Work out the finished part from the listing and answer in its coordinate system (mm). Coordinates: 2 decimals unless noted, no trailing zeros. Loops run counter-clockwise (first coordinate to the right, second up) from the corner with the lowest first, then second, coordinate; pieces in that order, holes last. Notation, with made-up numbers: M 64.5,29.25 L 117.5,29.25 A17 ccw 117.5,39.25 Z; hole C 7.25,-22 d3. An arc over 180 degrees is marked long. Write each question's results on one line, items separated by ' | '.
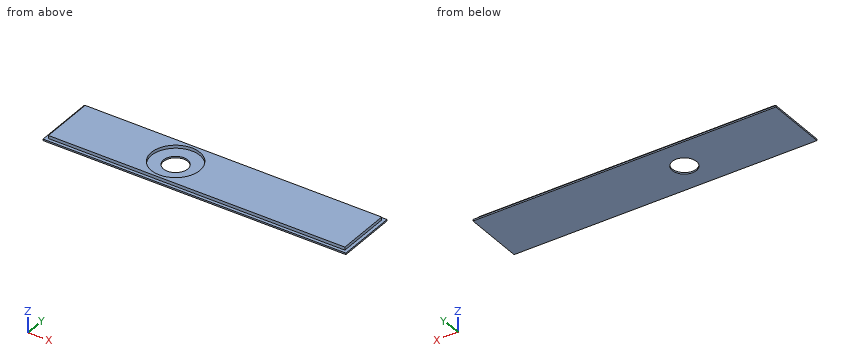
Autodesk Inventor part; units mm, degrees
ref_plane "YZ Plane" through (0, 0, 0) normal (1, 0, 0) x (0, 1, 0)
ref_plane "XZ Plane" through (0, 0, 0) normal (0, 1, 0) x (-1, 0, 0)
ref_plane "XY Plane" through (0, 0, 0) normal (0, 0, 1) x (1, 0, 0)
sketch "Boceto1" plane through (0, 0, 0) normal (0, 0, 1) x (1, 0, 0)
  line L0 (0, 0) -> (200, 0)
  line L1 (200, 0) -> (200, 40)
  line L2 (200, 40) -> (0, 40)
  line L3 (0, 40) -> (0, 0)
  circle A0 centre (74, 20) radius 8
  dimension "d0" = 200
  dimension "d1" = 40
  dimension "d2" = 16
  dimension "d3" = 74
  dimension "d4" = 20
extrude "Extrusión1" add sketch "Boceto1" along normal blind 1
sketch "Boceto2" plane through (0, 0, 1) normal (0, 0, 1) x (1, 0, 0)
  circle A0 centre (74, 20) radius 8
  line L0 (0, 0) -> (0, 40)
  line L1 (200, 0) -> (0, 0)
  line L2 (200, 40) -> (200, 0)
  line L3 (0, 40) -> (200, 40)
  line L4 (197.9, 37.9) -> (197.9, 2.1)
  line L5 (197.9, 2.1) -> (2.1, 2.1)
  line L6 (2.1, 2.1) -> (2.1, 37.9)
  line L7 (2.1, 37.9) -> (197.9, 37.9)
  circle A1 centre (74, 20) radius 16
  dimension "d7" = 2.1
  dimension "d8" = 32
extrude "Extrusión2" add sketch "Boceto2" along normal blind 2 contours L4 L5 L6 L7
properties part number "Tapa"
1) Straight lines are drawn through the part: probe 1 along Y at (x, z) = (74, 0.7); probe 2 along X at (y, z) = (20.5, 0.1); probe 3 along Y at (x, z) = (96.5, 2.7). For each, find the intervals that lie inside material, in ascending order. Write a range as [from, to].
Check result:
probe 1: [0, 12], [28, 40] | probe 2: [0, 66.02], [81.98, 200] | probe 3: [2.1, 37.9]
2) Find section D-D, the plane x = 105.5. Give the vertices of the cut face in (y, z), and give its area (3 significant figures).
Check result:
outline: M 0,0 L 40,0 L 40,1 L 37.9,1 L 37.9,3 L 2.1,3 L 2.1,1 L 0,1 Z | area: 112 mm^2
3) Find section A-A, the plane x = 74. Give the vertices of the cut face in (y, z).
Check result:
outline: M 0,0 L 12,0 L 12,1 L 4,1 L 4,3 L 2.1,3 L 2.1,1 L 0,1 Z; M 28,0 L 40,0 L 40,1 L 37.9,1 L 37.9,3 L 36,3 L 36,1 L 28,1 Z
4) Given pin 1 Ø2 at (x, y) = (77, 8.5) entering from +Z; pin 2 Ø1.6 at (y, z) = (13, 2) entering from +X; pin 3 Ø0.6 at (y, z) = (27, 2.5) entering from -X, each flat-ended and moving along its own axis, determine where each tip first touches the part or whether it passes through.
Check result:
pin 1: z = 1 | pin 2: x = 197.9 | pin 3: x = 2.1
5) Find section B-B, the plane y = 20. Give the vertices of the cut face in (x, z), and give its area (3 significant figures).
Check result:
outline: M 0,0 L 66,0 L 66,1 L 58,1 L 58,3 L 2.1,3 L 2.1,1 L 0,1 Z; M 82,0 L 200,0 L 200,1 L 197.9,1 L 197.9,3 L 90,3 L 90,1 L 82,1 Z | area: 512 mm^2
6) Find section C-C, the plane z = 0.5. Give the vertices of the cut face in (x, y).
Check result:
outline: M 0,0 L 200,0 L 200,40 L 0,40 Z; hole C 74,20 d16
